```python
from build123d import *

# Parameters (mm, degrees)
PAD004_DEPTH    = 17
PAD005_DEPTH    = 11
SKETCH007_R     = 11.1
POCKET001_DEPTH = 35
SKETCH015_R     = 2.05
POCKET003_DEPTH = 5


with BuildPart() as part:
    # Sketch005 → Pad004 (new body)
    with BuildSketch(Plane.YZ.offset(11)):
        with BuildLine():
            Line((-15, -29.6), (-101.569351, -29.6))
            Line((-101.569351, -29.6), (-101.569351, -0.4))
            Line((-101.569351, -0.4), (-15, -0.4))
            ThreePointArc((-15, -29.6), (-0.4, -15), (-15, -0.4))
        make_face()
    extrude(amount=PAD004_DEPTH)

    # Sketch006 → Pad005 (join)
    with BuildSketch(Plane.YZ):
        with BuildLine():
            ThreePointArc((-23.665016, -0.2), (-32.149529, -14.872954), (-23.883333, -29.67))
            Line((-101.569351, -29.67), (-23.883333, -29.67))
            Line((-101.569351, -0.2), (-101.569351, -29.67))
            Line((-23.665016, -0.2), (-101.569351, -0.2))
        make_face()
    extrude(amount=PAD005_DEPTH)

    # Sketch007 → Pocket001 (cut)
    with BuildSketch(Plane.YZ):
        with Locations((-15, -15)):
            Circle(SKETCH007_R)
    extrude(amount=POCKET001_DEPTH, mode=Mode.SUBTRACT)

    # Sketch015 → Pocket003 (cut)
    with BuildSketch(Plane.XY):
        with Locations((15, -92.5)):
            Circle(SKETCH015_R)
    extrude(amount=-POCKET003_DEPTH, mode=Mode.SUBTRACT)


solid = part.part
```
CAD build for the part. Positions are in the model's coordinates, mm. A direction names the side the tool comes from. Round coordinates to 2 decimals unless told otherwise and drop trailing zeros. Write each loop counter-clockwise with the first axis right and the second up, starting at its lowest first coordinate (ties: lowest second). Pieces come first, ordered by that corner, then holes. Notation, with made-up numbers: (63.25, -3.75) -> (116.25, -3.75) arc R32 ccw to (116.25, 32.25) -> close; hole circle Ø7 at (9, -28). An arc over 180 degrees is marked (long way). Answer in a Markdown table with one row per item. Add a question column.
Item 1: Saw through at C-C, the plane y = -92.5. Write the cut outline in (x, z).
Item 2: Drill centre lines: line 1 (Y direction, x = 17.5, z = -15); line 2 (Z direction, x = 20.5, y = -15); line 3 (Z direction, x = 19.75, y = -72.5). Where is each one in solid material? Low to high. Write a range as from..to.
Item 3: Saw through at B-B, the plane x = 15. Write the cut outline in (y, z).
Item 4: Saw through at A-A, the plane z = -15. Write the cut outline in (x, y).
Item 5: Drop flat-ended pins along their axis: pin 1 Ø3 at (y, z) = (-75.5, -20.5) entering from -X; pin 2 Ø13.5 at (y, z) = (-15, -15) entering from -X; pin 3 Ø3.5 at (x, y) = (14.5, -92) entering from +Z; pin 4 Ø14.5 at (y, z) = (-23.5, -17.5) entering from -X. Give the stop position or say it passes through.
Item 6: Saw through at D-D, the plane z = -10.5. Write the cut outline in (x, y), then the cut area to 3 significant figures.
Item 7: Which spindle directions (+Z, -Z, +X, -X, +Y, -Y) get a long thin tool onto all of the face, cutting with end or side? Do faces 1 (the face through (14.733, -90.467, -2.668)), 2 (the face through (5, -63, -29.67)). Say none if no direction does.
Item 8: Mould opens along Z. For faces 3 (the face through (5.423, -32.146, -14.625)), 4 (the face through (11, -27, -15)), 5 (the face through (19, -59, -0.4)), 6 (the face through (19, -58, -29.6)) say: pulls with the +Z half, pulls with the -Z half, needs draft (parallel to the pull), parting line crosses it, or undercut.
Findings below:
| question | item | result |
|---|---|---|
| 1 | outline | (0, -29.67) -> (11, -29.67) -> (11, -29.6) -> (28, -29.6) -> (28, -0.4) -> (17.05, -0.4) -> (17.05, -5) -> (12.95, -5) -> (12.95, -0.4) -> (11, -0.4) -> (11, -0.2) -> (0, -0.2) -> close |
| 2 | line 1 | y = -101.57..-26.1, -3.9..-0.4 |
| 2 | line 2 | z = -29.6..-26.1, -3.9..-0.4 |
| 2 | line 3 | z = -29.6..-0.4 |
| 3 | outline | (-101.57, -29.6) -> (-15, -29.6) arc R14.6 ccw to (-15, -0.4) -> (-90.45, -0.4) -> (-90.45, -5) -> (-94.55, -5) -> (-94.55, -0.4) -> (-101.57, -0.4) -> close; hole circle Ø22.2 at (-15, -15) |
| 4 | outline | (0, -101.57) -> (28, -101.57) -> (28, -26.1) -> (11, -26.1) -> (11, -32.15) -> (0, -32.15) -> close; (11, -3.9) -> (28, -3.9) -> (28, -0.4) -> (11, -0.4) -> close |
| 5 | pin 1 | stops at x = 0 |
| 5 | pin 2 | passes through |
| 5 | pin 3 | stops at z = -0.4 |
| 5 | pin 4 | stops at x = 11 |
| 6 | outline | (0, -101.57) -> (28, -101.57) -> (28, -25.15) -> (11, -25.15) -> (11, -31.55) -> (0, -31.55) -> close; (11, -4.85) -> (28, -4.85) -> (28, -1.11) -> (11, -1.11) -> close |
| 6 | area | 2,130 mm^2 |
| 7 | face 1 | +Z |
| 7 | face 2 | -Z, +X, -X, +Y, -Y |
| 8 | face 3 | undercut |
| 8 | face 4 | undercut |
| 8 | face 5 | pulls with the +Z half |
| 8 | face 6 | pulls with the -Z half |
